Part model, mm, in its own coordinate system. A direction names the side the tool comes from. Give positions to 0.01 mm unless a question says otherwise; leave off trailing zeros. Order: outer loops, then holes, each group sorted by start corner. A loop starts at its lowest first (then second) coordinate and runs counter-clockwise, first axis right, second up. Notation, with made-up numbers: M -38,-19 L 15,-19 A19 cw 15,17 Z; hole C -30.75,12.25 d5. An arc over 180 degrees is marked long. One line per question, with ' | ' between items.
```python
from build123d import *

# Parameters (mm, degrees)
SKETCH_1_R          = 1.75
EXTRUDE_1_DEPTH     = 2
FILLET_1_R          = 4
SKETCH_2_W          = 5
SKETCH_2_H          = 10
EXTRUDE_2_DEPTH     = 5
CUT_EXTRUDE_1_DEPTH = 0.2
SKETCH_5_W          = 18.176567436
SKETCH_5_H          = 8.683574631
EXTRUDE_3_DEPTH     = 5


with BuildPart() as part:
    # 草图1 → 凸台-拉伸1 (new body)
    with BuildSketch(Plane(origin=(0, 0, 0), x_dir=(1, 0, 0), z_dir=(0, 1, 0))):
        with BuildLine():
            Line((-34.475, 43.140944253), (34.475, 43.140944253))
            ThreePointArc((34.475, 43.140944253), (38.57, 39.045944253), (34.475, 34.950944253))
            Line((34.475, 34.950944253), (32.725, 33.200944253))
            Line((32.725, 33.200944253), (32.725, 13.200944253))
            Line((32.725, 13.200944253), (38.57, 7.355944253))
            Line((38.57, 7.355944253), (38.57, -9.759055747))
            Line((38.57, -9.759055747), (-38.57, -9.759055747))
            Line((-38.57, -9.759055747), (-38.57, 7.355944253))
            Line((-38.57, 7.355944253), (-32.725, 13.200944253))
            Line((-32.725, 13.200944253), (-32.725, 33.200944253))
            Line((-32.725, 33.200944253), (-34.475, 34.950944253))
            ThreePointArc((-34.475, 34.950944253), (-38.57, 39.045944253), (-34.475, 43.140944253))
        make_face()
        with Locations(Location((34.475, 39.045944253, 0), (0, 0, 270))):
            Circle(SKETCH_1_R, mode=Mode.SUBTRACT)
        with Locations(Location((34.475, -5.214055747, 0), (0, 0, 270))):
            Circle(SKETCH_1_R, mode=Mode.SUBTRACT)
        with Locations(Location((-34.475, -5.214055747, 0), (0, 0, 90))):
            Circle(SKETCH_1_R, mode=Mode.SUBTRACT)
        with Locations(Location((-34.475, 39.045944253, 0), (0, 0, 90))):
            Circle(SKETCH_1_R, mode=Mode.SUBTRACT)
    extrude(amount=EXTRUDE_1_DEPTH)

    # 圆角1
    fillet_1_edges = [part.edges().sort_by_distance(p)[0] for p in [
        (38.57, 1, 9.759055747),
        (-38.57, 1, 9.759055747),
    ]]
    fillet(fillet_1_edges, radius=FILLET_1_R)

    # 草图2 → 凸台-拉伸2 (add)
    with BuildSketch(Plane.XZ):
        with Locations((30.225, -29.368896619)):
            Rectangle(SKETCH_2_W, SKETCH_2_H)
        with Locations((-30.225, -27.845518443)):
            Rectangle(SKETCH_2_W, SKETCH_2_H)
        with Locations((30.225, -18.877356426)):
            Rectangle(SKETCH_2_W, SKETCH_2_H)
    extrude(amount=EXTRUDE_2_DEPTH)

    # 草图4 → 切除-拉伸1 (cut)
    with BuildSketch(Plane.XZ.offset(5)):
        Polygon((31.631043608, -19.986230369), (31.631043608, -17.932277654), (31.131043608, -17.932277654), (31.131043608, -18.656291548), (29.131043608, -18.656291548), (29.131043608, -17.932277654), (28.631043608, -17.932277654), (28.631043608, -19.986230369), (29.131043608, -19.986230369), (29.131043608, -19.151981589), (31.131043608, -19.151981589), (31.131043608, -19.986230369), align=None)
    extrude(amount=-CUT_EXTRUDE_1_DEPTH, mode=Mode.SUBTRACT)

    # 草图5 → 凸台-拉伸3 (add)
    with BuildSketch(Plane.XZ):
        with Locations((-22.049742487, -1.912133925)):
            Rectangle(SKETCH_5_W, SKETCH_5_H)
    extrude(amount=EXTRUDE_3_DEPTH)


solid = part.part
```
1. Slice it at C-C on x = -22. Give the cut face in (y, z), then the cut area to 3 significant figures.
Worked out:
outline: M -5,-6.25 L 0,-6.25 L 0,-43.14 L 2,-43.14 L 2,9.76 L 0,9.76 L 0,2.43 L -5,2.43 Z | area: 149 mm2
2. Slice it at A-A on y = -2. Give the cut face in (x, z) (3 decimals), then the cut area to 3 significant figures.
Worked out:
outline: M -32.725,-32.846 L -27.725,-32.846 L -27.725,-22.846 L -32.725,-22.846 Z; M -31.138,-6.254 L -12.961,-6.254 L -12.961,2.43 L -31.138,2.43 Z; M 27.725,-34.369 L 32.725,-34.369 L 32.725,-24.369 L 27.725,-24.369 Z; M 27.725,-23.877 L 32.725,-23.877 L 32.725,-13.877 L 27.725,-13.877 Z | area: 308 mm2
3. Probe L1, parallel to X at y = -0.75, z = -29 (3 decimals); L2, parallel to Y at x = 13, z = 1; L3, parallel to Z at x = -24.5, y = -3.75. List the from-to ranges inside material, lowest first. Write a range as from..to.
Worked out:
L1: x = -32.725..-27.725, 27.725..32.725 | L2: y = 0..2 | L3: z = -6.25..2.43
4. Drop flat-ended pins along their axis: pin 1 (4 mm diameter, centred on y = -2.5, z = -19, fed in from -X) (3 decimals); pin 2 (4 mm diameter, centred on x = -14.5, z = -36.5, fed in from -Y); pin 3 (1.5 mm diameter, centred on x = -18, y = -1.5, fed in from +Z). Give the stop position or say it passes through.
Worked out:
pin 1: stops at x = 27.725 | pin 2: stops at y = 0 | pin 3: stops at z = 2.43
5. Slice it at D-D on z = -4. Give the cut face in (x, y), then the cut area to 3 significant figures.
Worked out:
outline: M -38.57,0 L -31.14,0 L -31.14,-5 L -12.96,-5 L -12.96,0 L 38.57,0 L 38.57,2 L -38.57,2 Z | area: 245 mm2
6. Slice it at B-B on z = 5. Give the cut face in (x, y), then the cut area to 3 significant figures.
Worked out:
outline: M -38.57,0 L -36.21,0 L -36.21,2 L -38.57,2 Z; M -32.74,0 L 32.74,0 L 32.74,2 L -32.74,2 Z; M 36.21,0 L 38.57,0 L 38.57,2 L 36.21,2 Z | area: 140 mm2
7. Mould opens along X. For faces 5 (the flat face through (-12.961, -2, -2)), 6 (the flat face through (-31.138, -2, -2)), 7 (the cylindrical face through (32.767, 0.986, -39.425)) say: released by +X, released by -X, zero draft, split by the parting line, or undercut.
Worked out:
face 5: released by +X | face 6: released by -X | face 7: undercut
8. Tool access for faces 1 (the flat face through (-33.588, 0.986, -34.064)), 2 (the flat face through (-30, -2, -32.846)), 3 (the flat face through (33.612, 0.986, -34.088)), 4 (the flat face through (30, -2, -34.369)): list every direction of +Z, -Z, +X, -X, +Y, -Y with a clear straight run to the whole face (end or side of a thin tool).
Worked out:
face 1: -X, +Y, -Y | face 2: -Z, -X, -Y | face 3: +X, +Y, -Y | face 4: -Z, +X, -X, -Y
